Geometry check sheet. Reference: the model listing, model coordinates, mm. A direction names the side the tool comes from. Coordinates: 2 decimals unless noted, no trailing zeros. Write each loop counter-clockwise with the first axis right and the second up, starting at its lowest first coordinate (ties: lowest second). Pieces come first, ordered by that corner, then holes. Notation, with made-up numbers: (36.5, -22) -> (42.5, -22) arc R25 ccw to (42.5, 8) -> close; hole circle Ø6 at (-39.5, 89.25). An arc over 180 degrees is marked (long way). One line per question, with ' | ' between items.
from build123d import *

# Parameters (mm, degrees)
BOSS_EXTRUDE1_DEPTH = 20
CUT_EXTRUDE1_DEPTH  = 10
BOSS_EXTRUDE2_DEPTH = 30
CHAMFER1_SIZE       = 20
CHAMFER2_SIZE       = 20
CHAMFER2_SIZE2      = 30
SKETCH4_W           = 20
SKETCH4_H           = 20
BOSS_EXTRUDE3_DEPTH = 20
CUT_EXTRUDE2_DEPTH  = 10


with BuildPart() as part:
    # Sketch1 → Boss-Extrude1 (new body)
    with BuildSketch(Plane(origin=(0, 0, 0), x_dir=(1, 0, 0), z_dir=(0, 1, 0))):
        Polygon((0, 0), (60, 0), (60, -50), (50, -50), (50, -40), (40, -40), (30, -30), (10, -30), (10, -10), (0, -10), align=None)
    extrude(amount=BOSS_EXTRUDE1_DEPTH)

    # Sketch2 → Cut-Extrude1 (cut)
    with BuildSketch(Plane(origin=(0, 20, 0), x_dir=(1, 0, 0), z_dir=(0, 1, 0))):
        Polygon((30, -30), (10, -10), (10, -30), align=None)
    extrude(amount=-CUT_EXTRUDE1_DEPTH, mode=Mode.SUBTRACT)

    # Sketch3 → Boss-Extrude2 (add)
    with BuildSketch(Plane(origin=(0, 20, 0), x_dir=(1, 0, 0), z_dir=(0, 1, 0))):
        Polygon((0, 0), (60, 0), (60, -40), (40, -40), (40, -10), (10, -10), (0, -10), align=None)
    extrude(amount=BOSS_EXTRUDE2_DEPTH)

    # Chamfer1
    chamfer1_edges = [part.edges().sort_by_distance(p)[0] for p in [
        (50, 50, 40),
    ]]
    chamfer(chamfer1_edges, length=CHAMFER1_SIZE)

    # Chamfer2
    chamfer2_edges = [part.edges().sort_by_distance(p)[0] for p in [
        (0, 50, 5),
    ]]
    chamfer2_side = [part.faces().sort_by_distance(p)[0] for p in [
        (0, 25, 5),
    ]]
    chamfer(chamfer2_edges, length=CHAMFER2_SIZE, length2=CHAMFER2_SIZE2, reference=chamfer2_side[0])

    # Sketch4 → Boss-Extrude3 (add)
    with BuildSketch(Plane(origin=(0, 50, 0), x_dir=(1, 0, 0), z_dir=(0, 1, 0))):
        with Locations((50, -10)):
            Rectangle(SKETCH4_W, SKETCH4_H)
    extrude(amount=BOSS_EXTRUDE3_DEPTH)

    # Sketch5 → Cut-Extrude2 (cut)
    with BuildSketch(Plane(origin=(60, 0, 0), x_dir=(0, 0, -1), z_dir=(1, 0, 0))):
        Polygon((-20, 70), (-10, 70), (-20, 60), align=None)
    extrude(amount=-CUT_EXTRUDE2_DEPTH, mode=Mode.SUBTRACT)


solid = part.part
1. Cross-section at D-D on z = 25. Record the boundary of the cut face in (x, y), and give its area (3 significant figures).
Worked answers:
outline: (10, 0) -> (60, 0) -> (60, 45) -> (40, 45) -> (40, 20) -> (25, 20) -> (25, 10) -> (10, 10) -> close | area: 1,350 mm²
2. Cross-section at C-C on x = 35.5. Record the boundary of the cut face in (y, z), and give its area (3 significant figures).
Worked answers:
outline: (0, 0) -> (50, 0) -> (50, 10) -> (20, 10) -> (20, 35.5) -> (0, 35.5) -> close | area: 1,010 mm²
3. Material ranges on line 1 (Z direction, x = 43.5, y = 66.5); line 2 (X direction, y = 30, z = 17); line 3 (Y direction, x = 15, z = 25), recorded low to high. Write a range as from..to.
Worked answers:
line 1: 0..20 | line 2: 40..60 | line 3: 0..10
4. Mould release check, pull along Z, two halves, no side actions. Record for faces 6 (the face through (55, 65, 15)), 7 (the face through (55, 20, 45)): released by +Z, released by -Z, zero draft, split by the parting line, or undercut.
Worked answers:
face 6: released by +Z | face 7: zero draft
5. Go/stop test with flat-tipped pins: P1, Ø9, axis at x = 28, z = 23, coming from the +Y side; P2, Ø6, axis at x = 45, y = 63.5, coming from the +Z side; P3, Ø3, axis at y = 3.5, z = 18, coming from the -X side. Record where each tip stops, or that it passes through.
Worked answers:
P1: y = 20 | P2: z = 20 | P3: x = 10
6. Cross-section at A-A on z = 6. Record the boundary of the cut face in (x, y).
Worked answers:
outline: (0, 0) -> (60, 0) -> (60, 70) -> (40, 70) -> (40, 50) -> (30, 50) -> (0, 30) -> close
7. Cross-section at B-B on y = 5. Record the boundary of the cut face in (x, z), and give its area (3 significant figures).
Worked answers:
outline: (0, 0) -> (60, 0) -> (60, 50) -> (50, 50) -> (50, 40) -> (40, 40) -> (30, 30) -> (10, 30) -> (10, 10) -> (0, 10) -> close | area: 1,950 mm²
8. Tool access check on faces 1 (the face through (48, 58, 20)), 2 (the face through (55, 10, 50)), 3 (the face through (15, 10, 24)), 4 (the face through (50, 10, 45)), 5 (the face through (50, 67, 17)). Record the directions out of +Z, -Z, +X, -X, +Y, -Y that give a thin tool (end or side, any length) a straight path to the whole face; none if there is none.
Worked answers:
face 1: +Z, +X, -X, +Y | face 2: +Z, +X, -X, +Y, -Y | face 3: +Z, -X, +Y | face 4: +Z, -X, +Y, -Y | face 5: +Z, +X, +Y
